Autodesk Inventor part; units mm, degrees
ref_plane "YZ Plane" through (0, 0, 0) normal (1, 0, 0) x (0, 1, 0)
ref_plane "XZ Plane" through (0, 0, 0) normal (0, 1, 0) x (-1, 0, 0)
ref_plane "XY Plane" through (0, 0, 0) normal (0, 0, 1) x (1, 0, 0)
sketch "Sketch1" plane through (0, 0, 0) normal (0, 0, 1) x (1, 0, 0)
  circle A0 centre (0, 0) radius 6
  line L0 (0, 0) -> (0, 5)
  line L1 (0, 5) -> (3.3166, 5)
  line L2 (0, 5) -> (-3.3166, 5)
  line L3 (0, 0) -> (0, -5)
  line L4 (0, -5) -> (3.3166, -5)
  line L5 (0, -5) -> (-3.3166, -5)
  dimension "d0" = 12
  dimension "d1" = 5
  dimension "d2" = 5
extrude "Extrusion1" add sketch "Sketch1" along normal blind 15 contours A0 L4 L3 L0 L1 | L2 L0 L3 L5 A0
sketch "Sketch2" plane through (0, 0, 15) normal (0, 0, 1) x (1, 0, 0)
  arc A0 (-3.3166, 5) -> (-3.3166, -5) centre (0, 0) ccw
  line L0 (-6, 0) -> (-6, 4.5)
  line L1 (-5.5, 5) -> (5.5, 5)
  line L2 (6, 4.5) -> (6, -4.5)
  line L3 (5.5, -5) -> (-5.5, -5)
  line L4 (-6, -4.5) -> (-6, 5)
  arc A1 (-5.5, 5) -> (-6, 4.5) centre (-5.5, 4.5) ccw
  arc A2 (-6, -4.5) -> (-5.5, -5) centre (-5.5, -4.5) ccw
  arc A3 (5.5, -5) -> (6, -4.5) centre (5.5, -4.5) ccw
  arc A4 (6, 4.5) -> (5.5, 5) centre (5.5, 4.5) ccw
  point P0 (6, -5)
  point P1 (-6, -5)
  dimension "d5" = 12
  dimension "d6" = 0.5
  dimension "d32" = 10
  dimension "d33" = 5
extrude "Extrusion2" add sketch "Sketch2" along normal blind 1
sketch "Sketch3" plane through (0, 0, 16) normal (0, 0, 1) x (1, 0, 0)
  line L0 (0, 0) -> (-4, 0)
  line L1 (-4, 0) -> (-4, 3)
  line L2 (0, 0) -> (0, -3)
  line L3 (0, -3) -> (4, -3)
  circle A0 centre (-4, 3) radius 0.5
  circle A1 centre (4, -3) radius 0.5
  dimension "d9" = 4
  dimension "d10" = 3
  dimension "d11" = 3
  dimension "d12" = 4
  dimension "d13" = 1
  dimension "d14" = 1
extrude "Extrusion3" add sketch "Sketch3" along normal blind 2
sketch "Sketch4" plane through (-4, 3, 18) normal (0, 0, 1) x (1, 0, 0)
  line L0 (-1.5, 2) -> (9.5, 2)
  line L1 (10, 1.5) -> (10, -7.5)
  line L2 (9.5, -8) -> (-1.5, -8)
  line L3 (-2, -7.5) -> (-2, 1.5)
  arc A0 (-1.5, 2) -> (-2, 1.5) centre (-1.5, 1.5) ccw
  arc A1 (-2, -7.5) -> (-1.5, -8) centre (-1.5, -7.5) ccw
  arc A2 (9.5, -8) -> (10, -7.5) centre (9.5, -7.5) ccw
  arc A3 (10, 1.5) -> (9.5, 2) centre (9.5, 1.5) ccw
  line L4 (-1.5, -8) -> (9.5, -8)
  line L5 (-2, 1.5) -> (-2, -7.5)
  point P0 (4, -3)
  dimension "d17" = 0.5
  dimension "d36" = 10
  dimension "d37" = 12
  dimension "d38" = 0
  dimension "d39" = 0
extrude "Extrusion4" add sketch "Sketch4" along normal blind 1
sketch "Sketch5" plane through (-4, 3, 19) normal (0, 0, 1) x (1, 0, 0)
  circle A0 centre (0, 0) radius 0.5
  circle A1 centre (0, 0) radius 0.5
  circle A2 centre (8, -6) radius 0.5
  circle A3 centre (8, -6) radius 0.5
  point P0 (4, -3)
  point P1 (7.9, -5.5101)
  point P2 (7.9, -6.4899)
extrude "Extrusion5" add sketch "Sketch5" along normal blind 4
sketch "Sketch6" plane through (-4, 3, 23) normal (0, 0, 1) x (1, 0, 0)
  line L0 (-1.5, 2) -> (9.5, 2)
  line L1 (10, 1.5) -> (10, -7.5)
  line L2 (9.5, -8) -> (-1.5, -8)
  line L3 (-2, -7.5) -> (-2, 1.5)
  arc A0 (-1.5, 2) -> (-2, 1.5) centre (-1.5, 1.5) ccw
  arc A1 (10, 1.5) -> (9.5, 2) centre (9.5, 1.5) ccw
  arc A2 (9.5, -8) -> (10, -7.5) centre (9.5, -7.5) ccw
  arc A3 (-2, -7.5) -> (-1.5, -8) centre (-1.5, -7.5) ccw
  line L4 (-1.5, -8) -> (9.5, -8)
  line L5 (-2, 1.5) -> (-2, -7.5)
  point P0 (4, -3)
  dimension "d22" = 0.5
  dimension "d40" = 10
  dimension "d41" = 12
  dimension "d42" = 0
  dimension "d43" = 0
extrude "Extrusion6" add sketch "Sketch6" along normal blind 1
sketch "Sketch7" plane through (-4, 3, 24) normal (0, 0, 1) x (1, 0, 0)
  circle A0 centre (4, -3) radius 1.5
  line L0 (4, -3) -> (4, -2)
  line L1 (4, -2) -> (5.118, -2)
  line L2 (4, -2) -> (2.882, -2)
  dimension "d25" = 3
  dimension "d26" = 1
extrude "Extrusion7" add sketch "Sketch7" along normal blind 10 contours A0 L2 L1 picked at (3.9981, -3.6594)
sketch "Sketch8" plane through (0, 0, 0) normal (0, 0, -1) x (-1, 0, 0)
  circle A0 centre (0, 0) radius 5.95
  line L0 (0, 0) -> (0, -5)
  line L1 (3.3166, -5) -> (-3.3166, -5)
  line L2 (0, -5) -> (3.3166, -5)
  line L3 (3.3166, -5) -> (-3.2253, -5)
  line L4 (0, 0) -> (0, 5)
  line L5 (-3.3166, 5) -> (3.3166, 5)
  line L6 (3.289, 4.9583) -> (-3.289, 4.9583)
  point P0 (-3.2253, -5)
  point P1 (3.2253, -5)
  point P2 (3.2253, 5)
  point P3 (-3.2253, 5)
  dimension "d35" = 11.9
  dimension "d34" = 5
extrude "Extrusion8" add sketch "Sketch8" along normal blind 1 contours A0 L1 L0 L4 L6 | L6 L4 L5 A0 | L6 A0 L5 L4 | L4 L0 L1 A0 L6
sketch "Sketch9" plane through (0, 0, -1) normal (0, 0, -1) x (-1, 0, 0)
  arc A0 (-1.118, 1) -> (1.118, 1) centre (0, 0) ccw
  circle A1 centre (0, 0) radius 2.5
  dimension "d44" = 5
extrude "Extrusion9" add sketch "Sketch9" along normal blind 0.5
sketch "Sketch10" plane through (0, 0, -1.5) normal (0, 0, -1) x (-1, 0, 0)
  circle A0 centre (0, 0) radius 0.5
  dimension "d47" = 1
extrude "Extrusion10" add sketch "Sketch10" along normal blind 0.5
sketch "Sketch11" plane through (-4, 3, 24) normal (0, 0, 1) x (1, 0, 0)
  arc A0 (2.882, -2) -> (5.118, -2) centre (4, -3) ccw
  circle A1 centre (4, -3) radius 2
  dimension "d50" = 4
extrude "Extrusion11" add sketch "Sketch11" along normal blind 0.5
properties part number "minimotor"
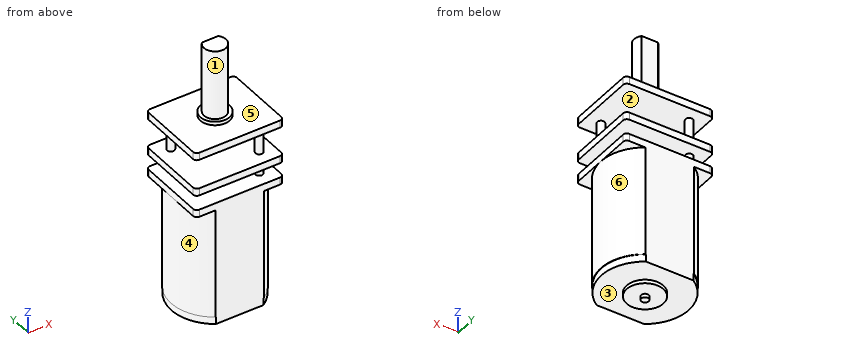
Check sheet for the modelled part. Datum: model origin and axes. Units: mm. Face numbers are marked on the shaded views. A direction names the side the tool comes from. Round coordinates to 2 decimals unless told otherwise and drop trailing zeros. Order: outer loops, then holes, each group sorted by start corner. A loop starts at its lowest first (then second) coordinate and runs counter-clockwise, first axis right, second up.
(1) Cross-section at B-B, the plane z = 21.5. Enter the section's corners in (x, y), and give its area (3 significant figures).
(2) Cross-section at D-D, the plane x = -4. Enter the section's corners in (y, z).
(3) Draft check along Z on the marked faces 1, 2 and 3. Enter one of: pulls with the +Z half, pulls with the -Z half, needs draft (parallel to the pull), parting line crosses it, or undercut.
(4) Cross-section at A-A, the plane x = 0. Enter the section's corners in (y, z).
(5) Scan lines: probe 1 along Z at (x, y) = (-3.25, 1.5); probe 2 along X at (y, z) = (0.25, 11); probe 3 along X at (y, z) = (1, 3). Record each from-to range of solid material in increasing order.
(6) Cross-section at C-C, the plane y = -3. Enter the section's corners in (x, z).
(7) Access from +Z, -Z, +X, -X, +Y, -Y to the whole of each face (thin tool, end or side, straight path). Record for the marked faces 4, 5 and 6.
(8) Go/stop test with flat-tipped pins: P1, Ø3, axis at x = 4.5, z = 29.5, coming from the +Y side; P2, Ø0.8, axis at x = 4, y = -1.5, coming from the -Z side; P3, Ø1.8, axis at x = -0.5, z = 28.5, coming from the +Y side. Record where each tip stops, or that it passes through.
Check sheet entries:
1. outline: circle Ø1 at (-4, 3); circle Ø1 at (4, -3)
1. area: 1.57 mm2
2. outline: (-5, 15) - (-4.47, 15) - (-4.47, 0) - (-4.4, 0) - (-4.4, -1) - (4.4, -1) - (4.4, 0) - (4.47, 0) - (4.47, 15) - (5, 15) - (5, 16) - (3.5, 16) - (3.5, 18) - (5, 18) - (5, 19) - (3.5, 19) - (3.5, 23) - (5, 23) - (5, 24) - (-5, 24) - (-5, 23) - (2.5, 23) - (2.5, 19) - (-5, 19) - (-5, 18) - (2.5, 18) - (2.5, 16) - (-5, 16) - close
3. face 1: needs draft
3. face 2: undercut
3. face 3: pulls with the -Z half
4. outline: (-5, -1) - (-2.5, -1) - (-2.5, -1.5) - (-0.5, -1.5) - (-0.5, -2) - (0.5, -2) - (0.5, -1.5) - (2.5, -1.5) - (2.5, -1) - (5, -1) - (5, 16) - (-5, 16) - close; (-5, 18) - (5, 18) - (5, 19) - (-5, 19) - close; (-5, 23) - (5, 23) - (5, 24) - (2, 24) - (2, 24.5) - (1, 24.5) - (1, 34) - (-1.5, 34) - (-1.5, 24.5) - (-2, 24.5) - (-2, 24) - (-5, 24) - close
5. probe 1: z = -1 to 16, 18 to 19, 23 to 24
5. probe 2: x = -5.99 to 5.99
5. probe 3: x = -5.92 to 5.92
6. outline: (-6, 15) - (-5.2, 15) - (-5.2, 0) - (-5.14, 0) - (-5.14, -1) - (5.14, -1) - (5.14, 0) - (5.2, 0) - (5.2, 15) - (6, 15) - (6, 16) - (4.5, 16) - (4.5, 18) - (6, 18) - (6, 19) - (4.5, 19) - (4.5, 23) - (6, 23) - (6, 24) - (-6, 24) - (-6, 23) - (3.5, 23) - (3.5, 19) - (-6, 19) - (-6, 18) - (3.5, 18) - (3.5, 16) - (-6, 16) - close
7. face 4: -Z, -X
7. face 5: +Z
7. face 6: -Z, +X
8. P1: passes through
8. P2: stops at z = -1
8. P3: stops at y = 1
